Check sheet for the modelled part. Datum: model origin and axes. Units: mm. A direction names the side the tool comes from. Give positions to 0.01 mm unless a question says otherwise; leave off trailing zeros. Write each loop counter-clockwise with the first axis right and the second up, starting at its lowest first coordinate (ties: lowest second). Pieces come first, ordered by that corner, then holes. Notation, with made-up numbers: M -14.75,52 L -0.75,52 A10 ccw -0.75,64 Z; hole C 74.25,52 d1. An arc over 180 degrees is marked long. Write item = value, one per line. Start each with the question number.
1) Cross-section at C-C, the plane z = -1. Record the cut outline in (x, y).
2) Cross-section at B-B, the plane x = 0. Record the cut outline in (y, z), plus the area to 3 significant figures.
3) Scan lines: line 1 along Y through (x, z) = (0, -12.75); line 2 along Y through (x, z) = (-5.25, -15.5); line 3 along X through (y, z) = (7, -13). Record each from-to range of solid material in increasing order. Write a range as [from, to].
4) Mould release check, pull along Y, two halves, no side actions. Record for faces 1 (the cylindrical face through (-1.73, -7.81, -7.15)), 2 (the cylindrical face through (-10.316, -7.91, 0.986)), 3 (the flat face through (0, 9, -9)), 4 (the flat face through (-2, -8, 4)): released by +Y, released by -Y, zero draft, split by the parting line, or undercut.
5) Cross-section at A-A, the plane y = 0. Record the cut outline in (x, z), plus the area to 3 significant figures.
6) Access from +Z, -Z, +X, -X, +Y, -Y to the whole of each face (thin tool, end or side, straight path). Record for faces 5 (the flat face through (-1, -10, 0)), 6 (the flat face through (0, -9, -9)), 7 (the cylindrical face through (-10.75, 0.15, -8.87)), 8 (the cylindrical face through (10.75, -0.15, -8.87)).
7) Go/stop test with flat-tipped pins: pin 1 (1.5 mm diameter, centred on y = -4.5, z = -1.5, fed in from +X); pin 2 (2 mm diameter, centred on x = -3.5, z = -7.5, fed in from +Y); pin 3 (10 mm diameter, centred on y = -7.5, z = -8, fed in from -X). Record where each tip stops, or that it passes through.
```python
from build123d import *

# Parameters (mm, degrees)
SKETCH1_R           = 13
SKETCH1_R_2         = 8
BOSS_EXTRUDE1_DEPTH = 4
BOSS_EXTRUDE2_DEPTH = 18
CUT_EXTRUDE1_START  = -18
SKETCH3_R           = 8
CUT_EXTRUDE1_DEPTH  = 18
CHAMFER1_SIZE       = 2


with BuildPart() as part:
    # Sketch1 → Boss-Extrude1 (new body)
    with BuildSketch(Plane.XY):
        Circle(SKETCH1_R)
        Circle(SKETCH1_R_2, mode=Mode.SUBTRACT)
    extrude(amount=BOSS_EXTRUDE1_DEPTH)

    # Sketch2 → Boss-Extrude2 (add)
    with BuildSketch(Plane(origin=(0, 0, 0), x_dir=(-1, 0, 0), z_dir=(0, 0, -1))):
        with BuildLine():
            Line((-5.878988008, 9), (5.878988008, 9))
            ThreePointArc((5.878988008, 9), (10.75, 0), (5.878988008, -9))
            Line((5.878988008, -9), (-5.878988008, -9))
            ThreePointArc((-5.878988008, -9), (-10.75, 0), (-5.878988008, 9))
        make_face()
    extrude(amount=BOSS_EXTRUDE2_DEPTH)

    # Sketch3 → Cut-Extrude1 (cut)
    with BuildSketch(Plane.XY.offset(CUT_EXTRUDE1_START)):
        Circle(SKETCH3_R)
    extrude(amount=CUT_EXTRUDE1_DEPTH, mode=Mode.SUBTRACT)

    # Chamfer1
    chamfer1_edges = [part.edges().sort_by_distance(p)[0] for p in [
        (-13, 0, 4),
    ]]
    chamfer(chamfer1_edges, length=CHAMFER1_SIZE)


solid = part.part
```
Reply:
q1.outline = M -5.88,-9 L 5.88,-9 A10.75 ccw 5.88,9 L -5.88,9 A10.75 ccw Z; hole C 0,0 d16
q2.outline = M -13,0 L -9,0 L -9,-18 L -8,-18 L -8,4 L -11,4 L -13,2 Z; M 8,-18 L 9,-18 L 9,0 L 13,0 L 13,2 L 11,4 L 8,4 Z
q2.area = 72.0 mm2
q3.line_1 = [-9, -8], [8, 9]
q3.line_2 = [-9, -6.04], [6.04, 9]
q3.line_3 = [-8.16, -3.87], [3.87, 8.16]
q4.face_1 = undercut
q4.face_2 = split by the parting line
q4.face_3 = released by +Y
q4.face_4 = zero draft
q5.outline = M -13,0 L -10.75,0 L -10.75,-18 L -8,-18 L -8,4 L -11,4 L -13,2 Z; M 8,-18 L 10.75,-18 L 10.75,0 L 13,0 L 13,2 L 11,4 L 8,4 Z
q5.area = 135 mm2
q6.face_5 = -Z
q6.face_6 = -Z, +X, -X, -Y
q6.face_7 = -Z, -X
q6.face_8 = -Z, +X
q7.pin_1 = 10.07
q7.pin_2 = 9
q7.pin_3 = -10.46
